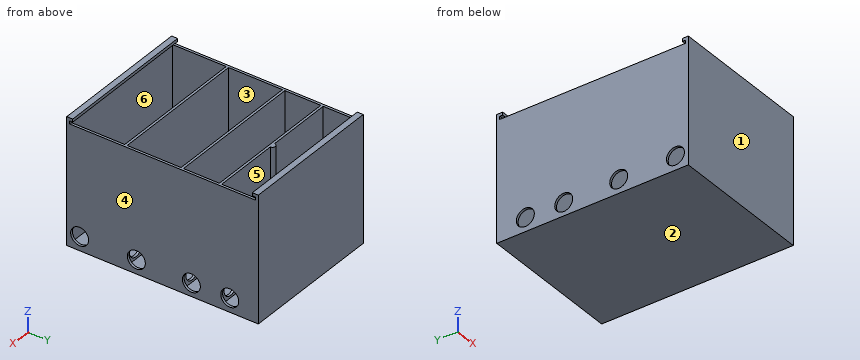
Autodesk Inventor part; units mm, degrees
ref_plane "YZ Plane" through (0, 0, 0) normal (1, 0, 0) x (0, 1, 0)
ref_plane "XZ Plane" through (0, 0, 0) normal (0, 1, 0) x (-1, 0, 0)
ref_plane "XY Plane" through (0, 0, 0) normal (0, 0, 1) x (1, 0, 0)
sketch "Sketch2" plane through (0, 0, 0) normal (0, 1, 0) x (-1, 0, 0)
  line L0 (0, 0) -> (152.4, 0)
  line L1 (152.4, 0) -> (152.4, -127)
  line L2 (152.4, -127) -> (0, -127)
  line L3 (0, -127) -> (0, 0)
  dimension "d2" = 152.4
  dimension "d3" = 127
extrude "Extrusion1" add sketch "Sketch2" along normal blind 2.54
sketch "Sketch3" plane through (0, 0, 0) normal (1, 0, 0) x (0, 0, -1)
  line L0 (127, 2.54) -> (0, 2.54)
  line L1 (0, 2.54) -> (127, 2.54)
  line L2 (127, 2.54) -> (127, 203.2)
  line L3 (127, 203.2) -> (0, 203.2)
  line L4 (0, 203.2) -> (0, 2.54)
  point P0 (0, 0)
  dimension "d6" = 127
  dimension "d7" = 200.66
extrude "Extrusion2" add sketch "Sketch3" against normal blind 2.54
sketch "Sketch4" plane through (-152.4, 0, -127) normal (-1, 0, 0) x (0, 0, 1)
  line L0 (0, 2.54) -> (127, 2.54)
  line L1 (127, 0) -> (127, 203.2)
  line L2 (0, 2.54) -> (127, 2.54)
  line L3 (127, 2.54) -> (127, 203.2)
  line L4 (127, 203.2) -> (0, 203.2)
  line L5 (0, 203.2) -> (0, 2.54)
extrude "Extrusion3" add sketch "Sketch4" against normal blind 2.54
sketch "Sketch5" plane through (0, 0, -127) normal (0, 0, -1) x (-1, 0, 0)
  line L0 (2.54, 2.54) -> (2.54, 203.2)
  line L1 (152.4, 203.2) -> (149.86, 203.2)
  line L2 (2.54, 2.54) -> (149.86, 2.54)
  line L3 (149.86, 2.54) -> (149.86, 203.2)
  line L4 (149.86, 203.2) -> (2.54, 203.2)
  line L5 (2.54, 203.2) -> (2.54, 2.54)
  point P0 (0, 0)
extrude "Extrusion4" add sketch "Sketch5" against normal blind 2.54
sketch "Sketch6" plane through (-152.4, 203.2, 0) normal (0, 1, 0) x (1, 0, 0)
  line L0 (0, 0) -> (2.54, 0)
  line L1 (149.86, 124.46) -> (2.54, 124.46)
  line L2 (2.54, 0) -> (149.86, 0)
  line L3 (149.86, 0) -> (149.86, 124.46)
  line L4 (149.86, 124.46) -> (2.54, 124.46)
  line L5 (2.54, 124.46) -> (2.54, 0)
  point P0 (152.4, 0)
extrude "Extrusion5" add sketch "Sketch6" against normal blind 2.54
sketch "Sketch7" plane through (-152.4, 0, 0) normal (0, 0, 1) x (1, 0, 0)
  line L0 (2.54, 200.66) -> (2.54, 2.54)
  line L1 (149.86, 200.66) -> (149.86, 2.54)
  line L2 (2.54, 59.69) -> (149.86, 59.69)
  line L3 (149.86, 59.69) -> (149.86, 62.23)
  line L4 (149.86, 62.23) -> (2.54, 62.23)
  line L5 (2.54, 62.23) -> (2.54, 59.69)
  line L6 (2.54, 119.38) -> (149.86, 119.38)
  line L7 (149.86, 119.38) -> (149.86, 121.92)
  line L8 (149.86, 121.92) -> (2.54, 121.92)
  line L9 (2.54, 121.92) -> (2.54, 119.38)
  line L10 (2.54, 160.02) -> (149.86, 160.02)
  line L11 (149.86, 160.02) -> (149.86, 162.56)
  line L12 (149.86, 162.56) -> (2.54, 162.56)
  line L13 (2.54, 162.56) -> (2.54, 160.02)
  dimension "d21" = 2.54
  dimension "d22" = 2.54
  dimension "d23" = 2.54
extrude "Extrusion6" add sketch "Sketch7" against normal blind 126.365 contours L12 L1 L10 L0 | L8 L1 L6 L0 | L4 L1 L2 L0
sketch "Sketch8" plane through (0, 0, 0) normal (1, 0, 0) x (0, 0, -1)
  point P0 (0, 0)
  point P1 (112.1689, 172.8914)
  point P2 (112.9467, 132.1734)
  point P3 (112.3284, 73.8307)
  point P4 (112.2777, 13.6778)
hole "Hole1" at (0, 172.8914, -112.1689) at (0, 132.1734, -112.9467) at (0, 73.8307, -112.3284) at (0, 13.6778, -112.2777) direction (-1, 0, 0) diameter 19.05 depth 201.6125 tip angle 126
sketch "Sketch9" plane through (-149.86, 162.56, 0) normal (0, 1, 0) x (1, 0, 0)
  point P0 (149.86, 0)
  point P1 (11.1706, 112.6616)
  point P2 (134.449, 112.5332)
hole "Hole2" at (-15.411, 162.56, -112.5332) at (-138.6894, 162.56, -112.6616) direction (0, -1, 0) diameter 19.05 depth 149.225 tip angle 126
sketch "Sketch10" plane through (-152.4, 0, 0) normal (0, 0, 1) x (1, 0, 0)
  line L0 (149.86, 162.56) -> (2.54, 162.56)
  arc A0 (79.375, 162.56) -> (73.025, 162.56) centre (76.2, 162.56) ccw
  point P0 (152.4, 0)
  dimension "d40" = 6.35
extrude "Extrusion7" add sketch "Sketch10" against normal blind 126.365
sketch "Sketch11" plane through (0, 0, 0) normal (1, 0, 0) x (0, 0, -1)
  line L0 (0, 0) -> (127, 0)
  line L1 (0, 0) -> (-6.35, 0)
  line L2 (-6.35, 0) -> (-6.35, 6.3374)
  line L3 (-6.35, 6.3374) -> (-3.175, 6.3374)
  line L4 (0, 6.3374) -> (0, 0)
  line L5 (0, 6.3374) -> (-3.175, 6.3374)
  line L6 (-3.175, 6.3374) -> (-3.175, 3.1687)
  line L7 (-3.175, 3.1687) -> (0, 3.1687)
  line L8 (0, 3.1687) -> (0, 6.3374)
  dimension "d43" = 6.35
extrude "Extrusion8" add sketch "Sketch11" against normal blind 152.4 contours L1 L2 L3 L6 L7 L4
sketch "Sketch13" plane through (0, 203.2, 0) normal (1, 0, 0) x (0, 0, -1)
  line L0 (0, -200.0313) -> (0, 0)
  line L1 (0, 0) -> (-6.35, 0)
  line L2 (-6.35, 0) -> (-6.35, -6.35)
  line L3 (-6.35, -6.35) -> (-3.175, -6.35)
  line L4 (0, -6.35) -> (0, 0)
  line L5 (0, -6.35) -> (-3.175, -6.35)
  line L6 (-3.175, -6.35) -> (-3.175, -3.175)
  line L7 (-3.175, -3.175) -> (0, -3.175)
  line L8 (0, -3.175) -> (0, -6.35)
  point P0 (0, -203.2)
  point P1 (0, -3.175)
  dimension "d50" = 6.35
  dimension "d51" = 6.35
extrude "Extrusion10" add sketch "Sketch13" against normal blind 152.4 contours L7 L6 L3 L2 L1 L0
properties part number "Shelf"
CAD build for the part. Positions are in the model's coordinates, mm. Face numbers are marked on the shaded views. A direction names the side the tool comes from. Coordinates: 2 decimals unless noted, no trailing zeros. Loops run counter-clockwise (first coordinate to the right, second up) from the corner with the lowest first, then second, coordinate; pieces in that order, holes last. Notation, with made-up numbers: (10, 70) -> (65, 70) arc R15 ccw to (65, 96) -> close; hole circle Ø7 at (57, -39.5). An arc over 180 degrees is marked (long way). One line per item, written item: value.
1. Slice it at D-D on y = 103. Write the cut outline in (x, z).
Answers:
outline: (-152.4, -127) -> (0, -127) -> (0, 0) -> (-2.54, 0) -> (-2.54, -124.46) -> (-149.86, -124.46) -> (-149.86, 0) -> (-152.4, 0) -> close
2. Drill centre lines: line 1 (Y direction, x = -128.5, z = -58); line 2 (X direction, y = 28, z = -57); line 3 (Y direction, x = -10, z = -118). Where is each one in solid material? Low to high. Write a range as [from, to].
Answers:
line 1: y = [0, 2.54], [59.69, 62.23], [119.38, 121.92], [160.02, 162.56], [200.66, 203.2]
line 2: x = [-152.4, -149.86], [-2.54, 0]
line 3: y = [0, 2.54], [200.66, 203.2]
3. Slice it at C-C on z = -92.5. Write the cut outline in (x, y) (3 decimals).
Answers:
outline: (-152.4, 0) -> (0, 0) -> (0, 203.2) -> (-152.4, 203.2) -> close; hole (-149.86, 2.54) -> (-2.54, 2.54) -> (-2.54, 59.69) -> (-149.86, 59.69) -> close; hole (-149.86, 62.23) -> (-2.54, 62.23) -> (-2.54, 119.38) -> (-149.86, 119.38) -> close; hole (-149.86, 121.92) -> (-2.54, 121.92) -> (-2.54, 160.02) -> (-149.86, 160.02) -> close; hole (-149.86, 162.56) -> (-79.375, 162.56) arc R3.175 cw to (-73.025, 162.56) -> (-2.54, 162.56) -> (-2.54, 200.66) -> (-149.86, 200.66) -> close
4. Which spindle directions (+Z, -Z, +X, -X, +Y, -Y) get a long thin tool onto all of the face, cutting with end or side? Do the marked faces 4, 5 and 6. Say none if no direction does.
Answers:
face 4: +Z, -Z, +X, +Y, -Y
face 5: +Z
face 6: none
5. Flat gauge pins, fed straight in: P1, Ø1.5, axis at x = -44, y = 151, coming from the +Z side; P2, Ø15, axis at y = 172.89, z = -112.17, coming from the +X side. Where does each tip first touch, or does it go through?
Answers:
P1: stops at z = -124.46
P2: stops at x = -74.76
6. Slice it at A-A on y = 168.5. Write the cut outline in (x, z), and give its area (3 significant figures).
Answers:
outline: (-152.4, -127) -> (0, -127) -> (0, -120.62) -> (-2.54, -120.62) -> (-2.54, -124.46) -> (-149.86, -124.46) -> (-149.86, -120.62) -> (-152.4, -120.62) -> close; (-152.4, -103.72) -> (-149.86, -103.72) -> (-149.86, 0) -> (-152.4, 0) -> close; (-2.54, -103.72) -> (0, -103.72) -> (0, 0) -> (-2.54, 0) -> close
area: 933 mm^2
7. Pull direction Y, two halves, no side cores. Call the marked faces 1, 2 and 3: pulls with the +Y half, pulls with the -Y half, needs draft (parallel to the pull), parting line crosses it, or undercut.
Answers:
face 1: pulls with the -Y half
face 2: needs draft
face 3: undercut
8. Slice it at B-B on x = -89. Write the cut outline in (y, z) (3 decimals).
Answers:
outline: (0, -127) -> (203.2, -127) -> (203.2, 6.35) -> (196.85, 6.35) -> (196.85, 3.175) -> (200.025, 3.175) -> (200.025, 0) -> (200.66, 0) -> (200.66, -124.46) -> (162.56, -124.46) -> (162.56, 0) -> (160.02, 0) -> (160.02, -124.46) -> (121.92, -124.46) -> (121.92, 0) -> (119.38, 0) -> (119.38, -124.46) -> (62.23, -124.46) -> (62.23, 0) -> (59.69, 0) -> (59.69, -124.46) -> (2.54, -124.46) -> (2.54, 0) -> (3.169, 0) -> (3.169, 3.175) -> (6.337, 3.175) -> (6.337, 6.35) -> (0, 6.35) -> close
